The drawing under review shows one solid part. Ordinate dimensions are in mm from its lowest x, y, z. A direction names the side the tool comes from. Coordinates: 2 decimals unless noted, no trailing zeros. Write each loop counter-clockwise with the first axis right and the second up, starting at its lowest first coordinate (ties: lowest second). Pieces come first, ordered by that corner, then holes.
Q1. Insertion check: pin 1 (11 mm diameter, centred on y = 5, z = 30.5, fed in from +X); pin 2 (4.5 mm diameter, centred on x = 5, y = 4, fed in from +Z); pin 3 (4.5 mm diameter, centred on x = 60.5, y = 56, fed in from +Z). Each pin has a flat end and moves straight along its axis. Give the tip position at first contact, or say it passes through.
Q2. For probe 1 along Y at (x, z) = (60, 25.5) (1 decimal); probe 2 along Z at (x, y) = (19.5, 66); probe 3 along Y at (x, z) = (54.5, 40) (1 decimal), list the stretches that pass through material, from the lowest coordinate up.
Q3. Machinability: for the marked faces 4, 5, 6 and 7, which of the approach directions +Z, -Z, +X, -X, +Y, -Y give a long, thin tool a straight path to every point of the face, cutting with its end or side? Answer none if there is none.
Q4. Take a section at D-D (z = 37.5). Give the boundary of the cut face in (x, y), and give its area (3 significant figures).
Q5. Mouldability with a two-part tool opening along X and no side actions: class the marked faces 1, 2 and 3 as pulls with the +X half, pulls with the -X half, needs draft (parallel to the pull), parting line crosses it, or undercut.
Q6. Take a section at C-C (x = 59.5). Give the boundary of the cut face in (y, z) (1 decimal), and give its area (3 significant figures).
Q7. Take a section at B-B (z = 23). Give the boundary of the cut face in (x, y) (1 decimal), and give its area (3 significant figures).
Q8. Take a section at A-A (y = 51). Give the boundary of the cut face in (x, z).
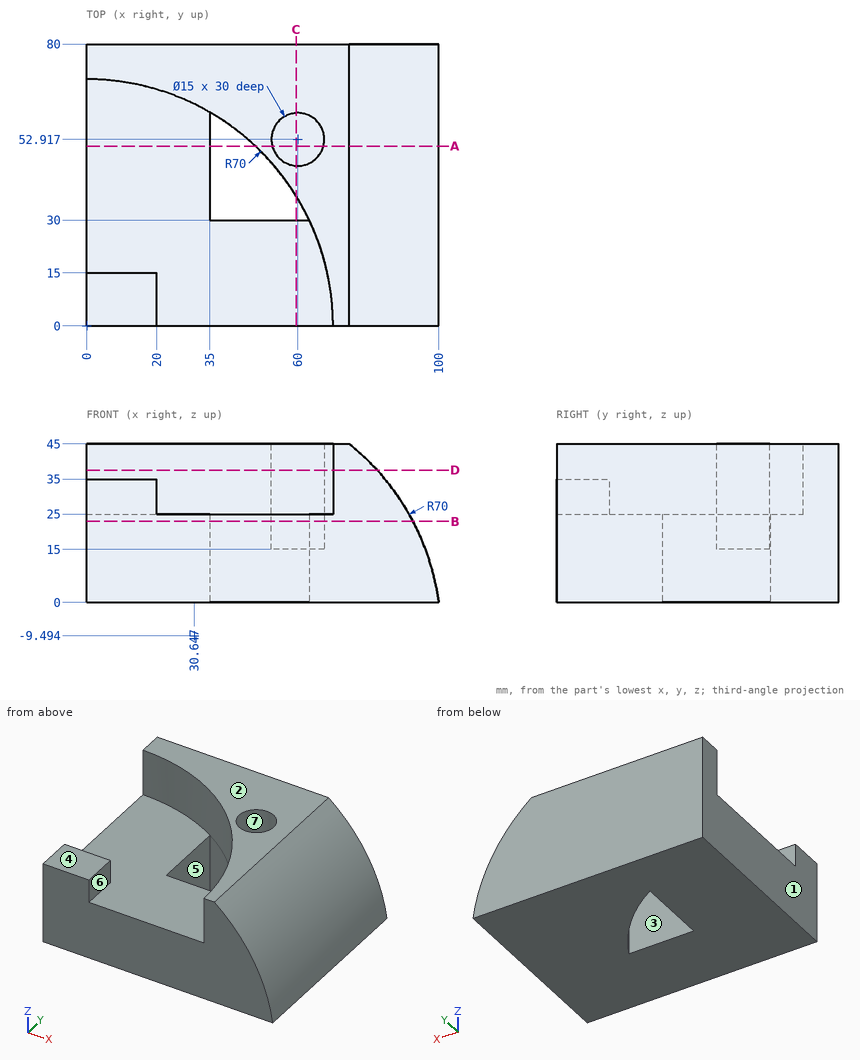
Response:
1. pin 1: stops at x = 91.56
1. pin 2: stops at z = 35
1. pin 3: stops at z = 15
2. probe 1: y = 36.1 to 45.4, 60.4 to 80
2. probe 2: z = 0 to 25
2. probe 3: y = 43.9 to 47.8, 58 to 80
3. face 4: +Z, -X, -Y
3. face 5: +Z, -Z
3. face 6: +Z, -Y
3. face 7: +Z
4. outline: (0, 70) arc R70 cw to (70, 0) - (82.53, 0) - (82.53, 80) - (0, 80) - close; hole circle Ø15 at (60, 52.92)
4. area: 2,580 mm2
5. face 1: pulls with the -X half
5. face 2: needs draft
5. face 3: undercut
6. outline: (0, 0) - (30, 0) - (30, 25) - (0, 25) - close; (36.9, 0) - (80, 0) - (80, 45) - (60.4, 45) - (60.4, 15) - (45.4, 15) - (45.4, 45) - (36.9, 45) - close
6. area: 2,240 mm2
7. outline: (0, 0) - (92.6, 0) - (92.6, 80) - (0, 80) - close; hole (35, 30) - (63.2, 30) arc R70 ccw to (35, 60.6) - close; hole circle Ø15 at (60, 52.9)
7. area: 6,710 mm2
8. outline: (0, 0) - (35, 0) - (35, 25) - (0, 25) - close; (47.95, 0) - (100, 0) arc R70 ccw to (74.58, 45) - (67.25, 45) - (67.25, 15) - (52.75, 15) - (52.75, 45) - (47.95, 45) - close
